Model file for the job. Use its own axes, mm. A direction names the side the tool comes from. Coordinates: 2 decimals unless noted, no trailing zeros. Order: outer loops, then holes, each group sorted by start corner. A loop starts at its lowest first (then second) coordinate and runs counter-clockwise, first axis right, second up. Notation, with made-up numbers: (53.25, -29) -> (61.25, -29) arc R21 cw to (61.25, -14) -> close; hole circle Ø5 at (-12.5, 77). An arc over 180 degrees is marked (long way). Return JSON: item names as keys, results as strings. Group by question number.
1) Cut at A-A (y = -4.5). Write the cut outline in (x, z).
2) Pull direction Y, two halves, no side cores. Call faces 1 (the flat face through (-67, 0, -38)), 2 (the flat face through (-68, -11, -153)), 3 (the cylindrical face through (-1.48, -9.17, -13.79)), 4 (the flat face through (-43, 3, -79)): +Y half, -Y half, draft (parallel to the pull), parting line (faces both ways), or undercut.
3) Cut at B-B (y = 4.5). Write the cut outline in (x, z), and give its area (3 significant figures).
4) Flat gauge pins, fed straight in: pin 1 (11 mm diameter, centred on y = -13, z = -51, fed in from -X); pin 2 (8 mm diameter, centred on x = -61, z = -47.5, fed in from -Y); pin 3 (9.5 mm diameter, centred on y = 10.5, z = -108, fed in from +X). Where does each tip first touch, or does it go through?
5) Probe line 1 (X direction, y = -13, z = -113); line 2 (X direction, y = -0.5, z = -44.5); line 3 (Z direction, x = -75, y = -2). List the from-to ranges inside material, lowest first.
6) Cut at D-D (z = -66). State how many separate pieces and enclosed holes the cut face has, and give its area (3 significant figures).
7) Which spindle directions (+Z, -Z, +X, -X, +Y, -Y) get a long thin tool onto all of the face, cutting with end or side? Do faces 5 (the flat face through (-33, -11, -79)), 6 (the flat face through (-17, -11, -73)), 7 (the cylindrical face through (-31.479, -11.775, -91.386)), 8 (the flat face through (-42.6, 0.2, -156)). Say none if no direction does.
8) Cut at C-C (x = -21). Write the cut outline in (y, z).
Autodesk Inventor part; units mm, degrees
ref_plane "YZ Plane" through (0, 0, 0) normal (1, 0, 0) x (0, 1, 0)
ref_plane "XZ Plane" through (0, 0, 0) normal (0, 1, 0) x (-1, 0, 0)
ref_plane "XY Plane" through (0, 0, 0) normal (0, 0, 1) x (1, 0, 0)
sketch "Sketch1" plane through (0, 0, 0) normal (0, 1, 0) x (-1, 0, 0)
  line L0 (0, 0) -> (84, 0)
  line L1 (84, 0) -> (84, -156)
  line L2 (84, -156) -> (0, -156)
  line L3 (0, -156) -> (0, 0)
  line L4 (84, 0) -> (84, -3)
  line L5 (84, -3) -> (81, -3) construction
  line L6 (0, -156) -> (0, -153)
  line L7 (0, -153) -> (3, -153) construction
  line L8 (81, -3) -> (3, -3)
  line L9 (3, -3) -> (3, -153)
  line L10 (3, -153) -> (81, -153)
  line L11 (81, -153) -> (81, -3)
  dimension "d0" = 84
  dimension "d1" = 156
  dimension "d2" = 3
  dimension "d3" = 3
  dimension "d4" = 3
  dimension "d5" = 3
extrude "Extrusion1" add sketch "Sketch1" along normal blind 15 contours L0 L1 L2 L3 | L11 L10 L9 L8
sketch "Sketch2" plane through (0, 15, 0) normal (0, 1, 0) x (1, 0, 0)
  line L0 (-84, 156) -> (-84, 0)
  line L1 (-84, 0) -> (-84, 3)
  line L2 (-84, 3) -> (-81, 3) construction
  line L3 (0, 0) -> (0, 156)
  line L4 (0, 156) -> (0, 153)
  line L5 (0, 153) -> (-3, 153) construction
  line L6 (-81, 3) -> (-3, 3)
  line L7 (-3, 3) -> (-3, 153)
  line L8 (-3, 153) -> (-81, 153)
  line L9 (-81, 153) -> (-81, 3)
  dimension "d8" = 3
  dimension "d9" = 3
  dimension "d10" = 3
  dimension "d11" = 3
extrude "Extrusion2" cut sketch "Sketch2" against normal blind 12
sketch "Sketch15" plane through (-81, 3, -3) normal (1, 0, 0) x (0, 0, -1)
  line L0 (87.2546, 33.7556) -> (153, 12)
  line L1 (153, 12) -> (150, 12)
  line L2 (153, 12) -> (-3, 12)
  line L3 (-3, 12) -> (153, 12)
  line L4 (-3, 12) -> (-3, 22)
  line L5 (87.2546, 33.7556) -> (-3, 22)
  dimension "d125" = 10
extrude "Extrusion12" add sketch "Sketch15" along normal blind 81 and the other way blind 3
sketch "Sketch16" plane through (0, 0, 0) normal (0, -1, 0) x (1, 0, 0)
  line L0 (0, -156) -> (-3, -156)
  line L1 (0, -153) -> (0, -156)
  line L2 (-3, -153) -> (-30, -153)
  line L3 (-30, -153) -> (-30, -83)
  line L4 (-30, -83) -> (-3, -83)
  line L5 (-3, -83) -> (-3, -153)
  line L6 (-81, -153) -> (-54, -153)
  line L7 (-54, -153) -> (-54, -83)
  line L8 (-54, -83) -> (-81, -83)
  line L9 (-81, -83) -> (-81, -153)
  line L10 (-3, -3) -> (-30, -3)
  line L11 (-30, -3) -> (-30, -73)
  line L12 (-30, -73) -> (-3, -73)
  line L13 (-3, -73) -> (-3, -3)
  line L14 (-81, -3) -> (-53.9385, -3)
  line L15 (-53.9385, -3) -> (-53.9385, -72.9998)
  line L16 (-53.9385, -72.9998) -> (-81, -72.9998)
  line L17 (-81, -72.9998) -> (-81, -3)
  line L18 (-33, -83) -> (-33, -80)
  line L19 (-33, -73) -> (-33, -76)
  line L20 (0, -156) -> (-33, -156)
  line L21 (-33, -156) -> (-33, -80)
  line L22 (0, -80) -> (0, -156)
  line L23 (-84, -156) -> (-51, -156)
  line L24 (-84, -80) -> (-84, -156)
  line L25 (0, 0) -> (-33, 0)
  line L26 (-33, 0) -> (-33, -76)
  line L27 (0, -76) -> (0, 0)
  line L28 (-84, 0) -> (-51, 0)
  line L29 (-51, 0) -> (-51, -72.9998)
  line L30 (-84, -76) -> (-84, 0)
  line L31 (-33, -80) -> (-33, -76)
  line L32 (0, -80) -> (0, -76)
  line L33 (0, -90.2546) -> (0, 0)
  line L34 (-51, -156) -> (-51, -83)
  line L35 (-51, -83) -> (-51, -72.9998)
  line L36 (-84, -80) -> (-84, -76)
  line L37 (-84, -156) -> (-84, 0)
extrude "Extrusion13" add sketch "Sketch16" along normal blind 22.5
sketch "Sketch17" plane through (0, -22.5, 0) normal (1, 0, 0) x (0, 0, -1)
  line L0 (156, 22.5) -> (0, 22.5)
  line L1 (0, 22.5) -> (16, 22.5)
  line L2 (16, 22.5) -> (16, 11.3)
  line L3 (156, 22.5) -> (156, 0)
  line L4 (156, 22.5) -> (140, 22.5)
  line L5 (140, 22.5) -> (140, 11.3)
  circle A0 centre (140, 11.3) radius 3
  circle A1 centre (16, 11.3) radius 3
  dimension "d152" = 16
  dimension "d153" = 11.2
  dimension "d154" = 16
  dimension "d155" = 11.2
  dimension "d156" = 6
  dimension "d157" = 6
extrude "Extrusion14" cut sketch "Sketch17" against normal blind 104.25
sketch "Sketch18" plane through (-30, 0, -3) normal (1, 0, 0) x (0, 0, -1)
  circle A0 centre (13, -11.2) radius 3
  line L0 (13, -11.2) -> (63, -11.2)
  circle A1 centre (63, -11.2) radius 1.5
  circle A2 centre (137, -11.2) radius 3
  line L1 (137, -11.2) -> (87, -11.2)
  circle A3 centre (87, -11.2) radius 1.5
  point P0 (-3, 0)
  dimension "d160" = 50
  dimension "d161" = 3
  dimension "d162" = 50
  dimension "d163" = 3
extrude "Extrusion15" cut sketch "Sketch18" against normal blind 35 contours A1 | A3
sketch "Sketch19" plane through (0, -22.5, 0) normal (1, 0, 0) x (0, 0, -1)
  line L0 (24.5867, 50.7024) -> (27.5867, 50.7024) construction
  line L1 (52.4457, 51.3057) -> (87.4417, 55.8638)
  line L2 (87.4417, 55.8638) -> (89.8555, 56.1782)
  line L3 (128.3377, 43.444) -> (89.8555, 56.1782)
  line L4 (128.3377, 43.444) -> (137.0302, 40.5676)
  line L5 (3, 37.5) -> (153, 37.5) construction
  line L6 (136.0152, 37.5) -> (139.0152, 37.5) construction
  line L7 (138.3236, 37.5) -> (141.3236, 37.5) construction
  line L8 (137.0302, 40.5676) -> (139.5212, 39.7465)
  line L9 (0, 47.5) -> (0, 0) construction
  line L10 (139.5212, 39.7465) -> (52.4457, 44.5852)
  line L11 (82.6373, 55.2381) -> (79.6624, 54.8506) construction
  line L12 (82.6373, 55.2381) -> (83.3756, 42.7599)
  line L13 (82.6373, 55.2381) -> (79.6624, 54.8506)
  line L14 (79.6624, 54.8506) -> (80.3616, 43.0339)
  line L15 (119.7308, 46.2922) -> (120.0541, 40.8283)
  line L16 (122.5789, 45.3497) -> (122.8556, 40.6726)
  line L17 (52.4457, 51.3057) -> (47.4876, 50.6599)
  line L18 (47.4876, 50.6599) -> (47.4876, 44.8607)
  line L19 (52.4457, 44.5852) -> (47.4876, 44.8607)
  point P0 (0, 22.5)
  point P1 (83.3692, 42.8668)
  dimension "d178" = 3
  dimension "d180" = 3
  dimension "d182" = 3
  dimension "d183" = 3
  dimension "d184" = 5
extrude "Extrusion17" cut sketch "Sketch19" against normal up to surface (84 mm away) contours L1 L14 L10 L19 L18 L17 | L1 L2 L3 L15 L10 L12 | L16 L3 L4 L8 L10
extrude "Extrusion18" add sketch "Sketch19" along normal blind 0.1 and the other way blind 84.1 contours L1 L14 L10 L19 L18 L17 | L1 L2 L3 L15 L10 L12 | L16 L3 L4 L8 L10
properties part number "prototype 2"
Answers below:
{
 "1": {"outline": "(-84, -156) -> (-51, -156) -> (-51, 0) -> (-84, 0) -> close; (-33, -156) -> (0, -156) -> (0, 0) -> (-33, 0) -> close; hole (-81, -153) -> (-54, -153) -> (-54, -83) -> (-81, -83) -> close; hole (-81, -73) -> (-53.94, -73) -> (-53.94, -3) -> (-81, -3) -> close; hole (-30, -153) -> (-3, -153) -> (-3, -83) -> (-30, -83) -> close; hole (-30, -73) -> (-3, -73) -> (-3, -3) -> (-30, -3) -> close"},
 "2": {"face 1": "-Y half", "face 2": "draft", "face 3": "undercut", "face 4": "undercut"},
 "3": {"outline": "(-84, -156) -> (0, -156) -> (0, 0) -> (-84, 0) -> close; hole (-81, -153) -> (-3, -153) -> (-3, -3) -> (-81, -3) -> close", "area": "1,400 mm^2"},
 "4": {"pin 1": "stops at x = -84", "pin 2": "stops at y = 0", "pin 3": "stops at x = 0"},
 "5": {"line 1": "x = -84 to -81, -54 to -51, -33 to -30, -3 to 0", "line 2": "x = -84 to -81, -53.94 to -51, -33 to -30, -3 to 0", "line 3": "z = -156 to -153, -83 to -73, -3 to 0"},
 "6": {"separate pieces": "3", "enclosed holes": "1", "area": "2,140 mm^2"},
 "7": {"face 5": "+Z, -Z, -Y", "face 6": "-Y", "face 7": "none", "face 8": "-Z, +X, -X, +Y, -Y"},
 "8": {"outline": "(-22.5, -156) -> (15, -156) -> (36.76, -90.25) -> (25, 0) -> (-22.5, 0) -> (-22.5, -3) -> (0, -3) -> (0, -73) -> (-22.5, -73) -> (-22.5, -83) -> (0, -83) -> (0, -153) -> (-22.5, -153) -> close; hole (3, -153) -> (15, -153) -> (15, -3) -> (3, -3) -> close"}
}
